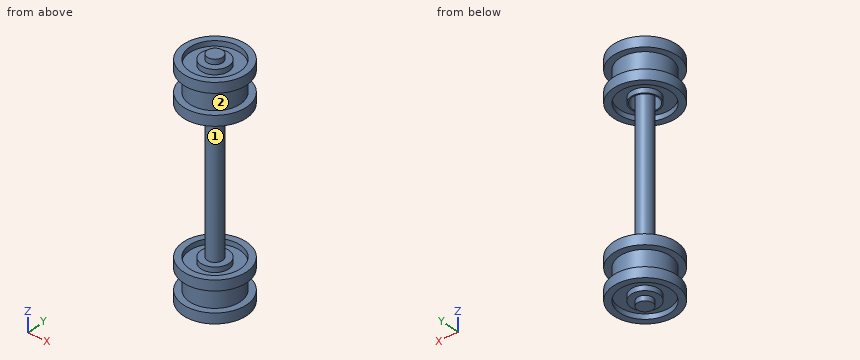
Autodesk Inventor part; units mm, degrees
ref_plane "Work Plane1" through (0, 0, 3.81) normal (0, 0, 1) x (1, 0, 0)
ref_plane "Work Plane2" through (0, 0, -19.05) normal (0, 0, -1) x (-1, 0, 0)
ref_plane "YZ Plane" through (0, 0, 0) normal (1, 0, 0) x (0, 1, 0)
sketch "Sketch3" plane through (0, 0, 0) normal (0, 0, 1) x (1, 0, 0)
  circle A0 centre (0, 0) radius 6.35
  dimension "d11" = 12.7
extrude "Extrusion3" add sketch "Sketch3" along normal blind 7.62
sketch "Sketch4" plane through (0, 0, 7.62) normal (0, 0, 1) x (1, 0, 0)
  circle A0 centre (0, 0) radius 7.9375
  circle A1 centre (0, 0) radius 6.35
  dimension "d14" = 15.875
  dimension "d15" = 12.7
extrude "Extrusion4" add sketch "Sketch4" along normal blind 1.27 and the other way blind 8.89
ref_plane "Work Plane1" through (0, 0, 3.81) normal (0, 0, 1) x (1, 0, 0)
sketch "Sketch5" plane through (0, 0, 3.81) normal (0, 0, 1) x (1, 0, 0)
  circle A0 centre (0, 0) radius 6.35
  circle A1 centre (0, 0) radius 8.89
  circle A2 centre (0, 0) radius 7.9375
  circle A3 centre (0, 0) radius 8.9298
extrude "Extrusion5" cut sketch "Sketch5" along normal mid plane 5.08 contours A2
sketch "Sketch6" plane through (0, 0, 7.62) normal (0, 0, 1) x (1, 0, 0)
  circle A0 centre (0, 0) radius 1.905
  circle A1 centre (0, 0) radius 3.4925
  dimension "d23" = 3.81
  dimension "d24" = 6.985
extrude "Extrusion6" add sketch "Sketch6" along normal blind 1.27 and the other way blind 8.89
sketch "Sketch7" plane through (0, 0, 7.62) normal (0, 0, 1) x (1, 0, 0)
  circle A0 centre (0, 0) radius 3.175
extrude "Extrusion7" cut sketch "Sketch7" against normal blind 9.2075
sketch "Sketch8" plane through (0, 0, 3.81) normal (0, 0, 1) x (1, 0, 0)
  circle A0 centre (0, 0) radius 1.905
  dimension "d36" = 3.81
extrude "Extrusion8" add sketch "Sketch8" along normal blind 6.35 and the other way blind 22.86
ref_plane "Work Plane2" through (0, 0, -19.05) normal (0, 0, -1) x (-1, 0, 0)
mirror "Mirror1" about plane through (0, 0, -19.05) normal (0, 0, -1) of "Extrusion5", "Extrusion4", "Extrusion3", "Extrusion8", "Extrusion6"
properties part number "Small Wheels for Polar Express [Copy]"
Verification items for the finished model (mm, model axes). Face numbers are marked on the shaded views. Round coordinates to 2 decimals unless told otherwise and drop trailing zeros. Order: outer loops, then holes, each group sorted by start corner. A loop starts at its lowest first (then second) coordinate and runs counter-clockwise, first axis right, second up. Notation, with made-up numbers: (36, 45.5) - (56, 45.5) arc R18 ccw to (56, 72.5) - close; hole circle Ø1 at (61.25, 28.25). An arc over 180 degrees is marked (long way). Use CSV: the item, a comma, the result in double quotes. Start each with the question number.
1) Section check A-A, the plane z = -28. Record the cut outline in (x, y) (3 decimals).
2) Go/stop test with flat-tipped pins: P1, Ø2, axis at y = -1.5, z = -12.5, coming from the -X side; P2, Ø5, axis at x = 3.5, y = -3.5, coming from the +Z side; P3, Ø2, axis at x = 1.5, z = -20.5, coming from the -Y side. Record where each tip stops, or that it passes through.
3) Thickness scan on L1, parallel to Y at x = 0, z = 8.65; L2, parallel to Z at x = -2.75, y = 7.25; L3, parallel to Y at x = 0, z = 0.75 (1 decimal). Record the ranges inside material, lowest first.
4) Mould release check, pull along X, two halves, no side actions. Record for the marked faces 1 and 2: +X half, -X half, draft (parallel to the pull), parting line (faces both ways), or undercut.
Answers:
1,outline,"circle Ø3.81 at (0, 0)"
2,P1,"stops at x = -1.84"
2,P2,"stops at z = 8.89"
2,P3,"stops at y = -1.84"
3,L1,"y = -7.94 to -6.35, -3.49 to 3.49, 6.35 to 7.94"
3,L2,"z = -46.99 to -44.45, -39.37 to -36.83, -1.27 to 1.27, 6.35 to 8.89"
3,L3,"y = -7.9 to -3.2, -1.9 to 1.9, 3.2 to 7.9"
4,face 1,"undercut"
4,face 2,"parting line"
